from build123d import *

# Parameters (mm, degrees)
SKETCH_1_R          = 22.75
EXTRUDE_1_DEPTH     = 4.2
SKETCH_2_R          = 16.5
EXTRUDE_2_DEPTH     = 18
SKETCH_3_R          = 12.5
CUT_EXTRUDE_1_DEPTH = 23.2
CHAMFER_1_SIZE      = 1


with BuildPart() as part:
    # 草图1 → 凸台-拉伸1 (new body)
    with BuildSketch(Plane.XY):
        Circle(SKETCH_1_R)
    extrude(amount=EXTRUDE_1_DEPTH)

    # 草图2 → 凸台-拉伸2 (add)
    with BuildSketch(Plane.XY.offset(4.2)):
        Circle(SKETCH_2_R)
    extrude(amount=EXTRUDE_2_DEPTH)

    # 草图3 → 切除-拉伸1 (cut, through all)
    with BuildSketch(Plane.XY.offset(22.2)):
        Circle(SKETCH_3_R)
    extrude(amount=-CUT_EXTRUDE_1_DEPTH, mode=Mode.SUBTRACT)

    # 倒角1
    chamfer_1_edges = [part.edges().sort_by_distance(p)[0] for p in [
        (-22.75, 0, 4.2),
        (-16.5, 0, 22.2),
    ]]
    chamfer(chamfer_1_edges, length=CHAMFER_1_SIZE)


solid = part.part
Design review of the part built by this model. Coordinates are the model's own, in mm. A direction names the side the tool comes from. Give positions to 0.01 mm unless a question says otherwise; leave off trailing zeros. Write each loop counter-clockwise with the first axis right and the second up, starting at its lowest first coordinate (ties: lowest second). Pieces come first, ordered by that corner, then holes. Notation, with made-up numbers: M -10,3 L 34,3 A26 ccw 34,17 Z; hole C 72.25,5.5 d2. An arc over 180 degrees is marked long. Return JSON: item names as keys, results as strings. Group by question number.
Item 1: Take a section at C-C (z = 5.5). Give the boundary of the cut face in (x, y).
Item 2: Tool access review of faces 1 (the flat face through (1, 13, 22.2)), 2 (the flat face through (8, 15, 4.2)): name each direction out of +Z, -Z, +X, -X, +Y, -Y from which nothing blocks a thin tool from reaching the whole face with its end or side.
Item 3: The part is to be moulded in two halves that separate along X. For faces 3 (the flat face through (10, -10, 0)), 4 (the cylindrical face through (-18.054, -13.843, 1.578)), 5 (the cylindrical face through (11.923, 3.755, 11.255)), say which applies: pulls with the +X half, pulls with the -X half, needs draft (parallel to the pull), parting line crosses it, or undercut.
Item 4: Wall thickness on line 1 along Y through (x, z) = (0, 12.5); line 2 along Z through (x, y) = (-9, -14.5); line 3 along Y through (x, z) = (-2, 15.75): over which ranges is each line inside the solid? List them lowest first.
Item 5: Take a section at A-A (y = 0). Give the boundary of the cut face in (x, z), plus the area to 3 significant figures.
Item 6: Clearance check with flat-ended pins moving along their axes: pin 1 Ø5 at (x, y) = (-8, -2.5) entering from +Z; pin 2 Ø4 at (y, z) = (-5.5, 11) entering from -X; pin 3 Ø1 at (x, z) = (12.5, 5.5) entering from +Y; pin 4 Ø3 at (x, z) = (14.5, 5.5) entering from +Y. State where each tip first meets the part, or that it passes through.
Return value:
{
 "1": {"outline": "C 0,0 d33; hole C 0,0 d25"},
 "2": {"face 1": "+Z, +X, -X, +Y, -Y", "face 2": "+Z"},
 "3": {"face 3": "needs draft", "face 4": "parting line crosses it", "face 5": "undercut"},
 "4": {"line 1": "y = -16.5 to -12.5, 12.5 to 16.5", "line 2": "z = 0 to 4.2", "line 3": "y = -16.38 to -12.34, 12.34 to 16.38"},
 "5": {"outline": "M -22.75,0 L -12.5,0 L -12.5,22.2 L -15.5,22.2 L -16.5,21.2 L -16.5,4.2 L -21.75,4.2 L -22.75,3.2 Z; M 12.5,0 L 22.75,0 L 22.75,3.2 L 21.75,4.2 L 16.5,4.2 L 16.5,21.2 L 15.5,22.2 L 12.5,22.2 Z", "area": "228 mm2"},
 "6": {"pin 1": "passes through", "pin 2": "stops at x = -16.12", "pin 3": "stops at y = 11.32", "pin 4": "stops at y = 16.85"}
}
